```python
from build123d import *

# Parameters (mm, degrees)
F1_DEPTH = 12.7
F2_R     = 6.95662
F3_DEPTH = 3.175
F5_DEPTH = 3.175


with BuildPart() as f1:
    # F0 (on Top) → F1 (new body)
    with BuildSketch(Plane.XY):
        with BuildLine():
            ThreePointArc((-31.390282, 21.59306), (-11.305757, -36.383923), (38.1, 0))
            ThreePointArc((38.1, 0), (36.383923, 11.305757), (31.390282, 21.59306))
            ThreePointArc((31.390282, 21.59306), (23.24256, 30.189293), (12.848724, 35.868096))
            ThreePointArc((12.848724, 35.868096), (0, 38.1), (-12.848724, 35.868096))
            ThreePointArc((-12.848724, 35.868096), (-23.24256, 30.189293), (-31.390282, 21.59306))
        make_face()
        with BuildLine():
            ThreePointArc((12.848724, 35.868096), (23.24256, 30.189293), (31.390282, 21.59306))
            ThreePointArc((31.390282, 21.59306), (33.31594, 43.273405), (12.848724, 35.868096))
        make_face()
        with BuildLine():
            ThreePointArc((-12.848724, 35.868096), (-33.31594, 43.273405), (-31.390282, 21.59306))
            ThreePointArc((-31.390282, 21.59306), (-23.24256, 30.189293), (-12.848724, 35.868096))
        make_face()
    extrude(amount=-F1_DEPTH)

    # F2 (on face) → F3 (join)
    with BuildSketch(Plane.XY):
        with Locations((-16.985364, 20.710224)):
            Circle(F2_R)
        with Locations((16.985364, 20.710224)):
            Circle(F2_R)
    extrude(amount=F3_DEPTH)

    # F4 (on face) → F5 (cut)
    with BuildSketch(Plane.XY):
        with BuildLine():
            Line((-32.182794, 30.543854), (-19.965252, 37.397597))
            ThreePointArc((-19.965252, 37.397597), (-30.11931, 41.18189), (-32.182794, 30.543854))
        make_face()
        with BuildLine():
            ThreePointArc((32.182794, 30.543854), (30.11931, 41.18189), (19.965252, 37.397597))
            Line((19.965252, 37.397597), (32.182794, 30.543854))
        make_face()
    extrude(amount=-F5_DEPTH, mode=Mode.SUBTRACT)


solid = f1.part
```
Could you check a few things on this model? Use its own coordinates, in mm. A direction names the side the tool comes from. Coordinates: 2 decimals unless noted, no trailing zeros. Write each loop counter-clockwise with the first axis right and the second up, starting at its lowest first coordinate (ties: lowest second). Pieces come first, ordered by that corner, then holes. Notation, with made-up numbers: (-12.5, 51.25) -> (19.5, 51.25) arc R5 ccw to (19.5, 59.25) -> close; hole circle Ø8 at (76.5, 21.25). An arc over 180 degrees is marked (long way). Return JSON: item names as keys, results as strings.
(1) Imagine slicing it at D-D, the plane x = 27. Please give me the cut outline in (y, z) (3 decimals), then the cut area to 3 significant figures.
Numbers:
{"outline": "(-26.881, -12.7) -> (45.859, -12.7) -> (45.859, 0) -> (42.081, 0) -> (42.081, -3.175) -> (33.451, -3.175) -> (33.451, 0) -> (-26.881, 0) -> close", "area": "896 mm2"}
(2) Imagine slicing it at A-A, the plane z = -2.25. Please give me the cut outline in (x, y).
Numbers:
{"outline": "(-31.39, 21.59) arc R38.1 ccw (long way) to (38.1, 0) arc R38.1 ccw to (31.39, 21.59) arc R12.91 ccw (long way) to (12.85, 35.87) arc R38.1 ccw to (-12.85, 35.87) arc R12.91 ccw (long way) to start; hole (-32.18, 30.54) -> (-19.97, 37.4) arc R7.1 ccw (long way) to start; hole (19.97, 37.4) -> (32.18, 30.54) arc R7.1 ccw (long way) to start"}
(3) I'm going to push flat-ended pins straight in: pin 1 (6 mm diameter, centred on x = 26, y = 34, fed in from +Z); pin 2 (2 mm diameter, centred on y = -11, z = -8.5, fed in from +X); pin 3 (6 mm diameter, centred on x = -3.5, z = -7.5, fed in from +Y). Where does each tip first touch, or does it pass through?
Numbers:
{"pin 1": "stops at z = 0", "pin 2": "stops at x = 36.76", "pin 3": "stops at y = 38.1"}
(4) I need wall thicknesses on L1, parallel to Y at x = -33, z = -1.5; L2, parallel to Z at x = 23.5, y = -22; L3, parallel to Y at x = -32.5, z = -2. Which ranges of each line are inside material? Lowest first, please.
Numbers:
{"L1": "y = -19.04 to 19.04, 22.58 to 31.82, 38.16 to 43.51", "L2": "z = -12.7 to 0", "L3": "y = -19.88 to 19.88, 22.24 to 30.97, 39.01 to 43.85"}
(5) Imagine slicing it at B-B, the plane x = 0. Please give me the cut outline in (y, z).
Numbers:
{"outline": "(-38.1, -12.7) -> (38.1, -12.7) -> (38.1, 0) -> (-38.1, 0) -> close"}
(6) Imagine slicing it at C-C, the plane y = 26.5. Please give me the cut outline in (x, z) (3 decimals), then the cut area to 3 significant figures.
Numbers:
{"outline": "(-36.565, -12.7) -> (36.565, -12.7) -> (36.565, 0) -> (20.842, 0) -> (20.842, 3.175) -> (13.129, 3.175) -> (13.129, 0) -> (-13.129, 0) -> (-13.129, 3.175) -> (-20.842, 3.175) -> (-20.842, 0) -> (-36.565, 0) -> close", "area": "978 mm2"}
(7) We'd pull the mould along X, two halves only. Please class faces 3 (the flat face through (-1, 5, -12.7)), 4 (the cylindrical face through (-22.51, 16.48, 1.57)): +X half, -X half, draft (parallel to the pull), parting line (faces both ways), or undercut.
Numbers:
{"face 3": "draft", "face 4": "undercut"}
(8) Which directions (+Z, -Z, +X, -X, +Y, -Y) give clear straight access to the entire face, cutting with the end or side of a thin tool? Please do faces 1 (the cylindrical face through (33.6, 43.05, -6.26)), 2 (the cylindrical face through (-29.968, 41.264, -1.565)).
Numbers:
{"face 1": "+Z, -Z", "face 2": "+Z"}
